Autodesk Inventor part; units mm, degrees
ref_plane "YZ Plane" through (0, 0, 0) normal (1, 0, 0) x (0, 1, 0)
ref_plane "XZ Plane" through (0, 0, 0) normal (0, 1, 0) x (-1, 0, 0)
ref_plane "XY Plane" through (0, 0, 0) normal (0, 0, 1) x (1, 0, 0)
sketch "Boceto1" plane through (0, 0, 0) normal (0, 1, 0) x (-1, 0, 0)
  line L0 (13.5057, -0.2828) -> (-21.8496, -35.6382)
  line L1 (13.5057, -0.2828) -> (-0.2828, 13.5057)
  line L2 (-0.2828, 13.5057) -> (-35.6382, -21.8496)
  line L3 (-35.6382, -21.8496) -> (-21.8496, -35.6382)
  circle A0 centre (12.6395, 5.7452) radius 1.65
  circle A1 centre (5.7452, 12.6395) radius 1.65
  circle A2 centre (-27.312, -34.2063) radius 1.65
  circle A3 centre (-34.2063, -27.312) radius 1.65
  arc A4 (14.2895, -13.2687) -> (-9.4509, 17.0567) centre (0, 0) ccw
  line L4 (-40.2344, 0) -> (-9.4509, 17.0567)
  line L5 (-40.2344, 0) -> (-43.2344, 0)
  line L6 (-19.0256, -57) -> (14.2895, -13.2687)
  line L7 (-43.2344, -57) -> (-19.0256, -57)
  line L8 (-43.2344, 0) -> (-47.2344, 0)
  line L9 (-47.2344, 0) -> (-47.2344, -14)
  line L10 (-47.2344, -14) -> (-43.2344, -14)
  line L11 (-43.2344, -57) -> (-47.2344, -57)
  line L12 (-47.2344, -57) -> (-47.2344, -43)
  line L13 (-47.2344, -43) -> (-43.2344, -43)
  line L14 (-47.2344, -21.5) -> (-43.2344, -21.5)
  line L15 (-47.2344, -21.5) -> (-47.2344, -35.5)
  line L16 (-47.2344, -35.5) -> (-43.2344, -35.5)
  line L17 (-43.2344, -14) -> (-43.2344, -21.5)
  line L18 (-43.2344, -35.5) -> (-43.2344, -43)
  dimension "d17" = 3
  dimension "d21" = 14
  dimension "d22" = 14
  dimension "d25" = 14
  dimension "d109" = 7.5
  dimension "d110" = 7.5
  dimension "d111" = 4
  dimension "d112" = 57
extrude "Extrusión1" add sketch "Boceto1" along normal blind 3
properties part number "planos robot"
Can you work these out from the model? Positions are in its coordinate system, mm. A direction names the side the tool comes from. Coordinates: 2 decimals unless noted, no trailing zeros. Write each loop counter-clockwise with the first axis right and the second up, starting at its lowest first coordinate (ties: lowest second). Pieces come first, ordered by that corner, then holes. Notation, with made-up numbers: (81, 42.25) - (115, 42.25) arc R9 cw to (115, 55.25) - close; hole circle Ø2 at (27.5, 53). An arc over 180 degrees is marked (long way). Return JSON: item names as keys, results as strings. Group by question number.
Item 1: If we section it at B-B (z = -9): Write out the boundary of the cut face in (x, y), then the cut area to 3 significant figures.
Item 2: If we section it at D-D (y = 2.1): Write out the boundary of the cut face in (x, z), then the cut area to 3 significant figures.
Item 3: Which directions (+Z, -Z, +X, -X, +Y, -Y) give clear straight access to the entire face, cutting with the end or side of a thin tool? Please do faces 1 (the face through (45, 1, -43)), 2 (the face through (3.92, 1.48, -17.71)), 3 (the face through (44, 1, 0)).
Item 4: If we section it at A-A (x = -5.5): Write out the boundary of the cut face in (y, z), then the cut area to 3 significant figures.
Item 5: Please list where these lines run through material, in increasing order: probe 1 along Z at (x, y) = (33, 0.2); probe 2 along Z at (x, y) = (22.5, 2.6); probe 3 along X at (y, z) = (0.35, -26.5).
Item 6: If we section it at C-C (x = 2): Write out the boundary of the cut face in (y, z).
Item 7: We'd pull the mould along X, two halves only. Please class faces 4 (the face through (45, 1, -14)), 5 (the face through (17.71, 1.48, -3.92)), 6 (the face through (47.234, 1, -28)): pulls with the +X half, pulls with the -X half, needs draft (parallel to the pull), parting line crosses it, or undercut.
Item 8: I'm going to push flat-ended pins straight in: pin 1 Ø1.5 at (x, y) = (46, 2) entering from +Z; pin 2 Ø1.5 at (x, y) = (-8.5, 1) entering from -Z; pin 3 Ø1 at (y, z) = (1, -16.5) entering from -X. Where does each tip first touch, or does it pass through?
Return value:
{
 "1": {"outline": "(-17.3, 0) - (-4.79, 0) - (-4.79, 3) - (-17.3, 3) - close; (22.79, 0) - (47.23, 0) - (47.23, 3) - (22.79, 3) - close", "area": "111 mm^2"},
 "2": {"outline": "(-14.29, -13.27) - (19.03, -57) - (47.23, -57) - (47.23, -43) - (43.23, -43) - (43.23, -35.5) - (47.23, -35.5) - (47.23, -21.5) - (43.23, -21.5) - (43.23, -14) - (47.23, -14) - (47.23, 0) - (40.23, 0) - (9.45, 17.06) arc R19.5 ccw to start; hole circle Ø3.3 at (-12.64, 5.75); hole (-13.51, -0.28) - (21.85, -35.64) - (35.64, -21.85) - (0.28, 13.51) - close; hole circle Ø3.3 at (-5.75, 12.64); hole circle Ø3.3 at (27.31, -34.21); hole circle Ø3.3 at (34.21, -27.31)", "area": "2,490 mm^2"},
 "3": {"face 1": "+X, +Y, -Y", "face 2": "+Y, -Y", "face 3": "+Z, +X, +Y, -Y"},
 "4": {"outline": "(0, -24.81) - (3, -24.81) - (3, -8.29) - (0, -8.29) - close; (0, 7.72) - (3, 7.72) - (3, 11.01) - (0, 11.01) - close; (0, 14.27) - (3, 14.27) - (3, 18.71) - (0, 18.71) - close", "area": "72.7 mm^2"},
 "5": {"probe 1": "z = -57 to -28.44, -26.19 to -24.49, -19.21 to 4.01", "probe 2": "z = -57 to -34.99, -8.71 to 9.83", "probe 3": "x = -4.21 to 12.71, 30.99 to 32.77, 35.64 to 47.23"},
 "6": {"outline": "(0, -34.65) - (3, -34.65) - (3, -15.79) - (0, -15.79) - close; (0, 11.79) - (3, 11.79) - (3, 19.4) - (0, 19.4) - close"},
 "7": {"face 4": "needs draft", "face 5": "undercut", "face 6": "pulls with the +X half"},
 "8": {"pin 1": "stops at z = 0", "pin 2": "stops at z = -21.85", "pin 3": "stops at x = -12.21"}
}
